from build123d import *

# Parameters (mm, degrees)
F0_W      = 50.8
F0_H      = 152.4
F1_DEPTH  = 914.4
F3_DEPTH  = 25.4
F5_DEPTH  = 914.401
F7_DEPTH  = 914.401
F9_DEPTH  = 50.801
F11_DEPTH = 27.94


with BuildPart() as f1:
    # F0 (on Right) → F1 (new body)
    with BuildSketch(Plane.YZ):
        with Locations((-25.4, 49.212513)):
            Rectangle(F0_W, F0_H)
    extrude(amount=F1_DEPTH)

    # F2 (on face) → F3 (cut)
    with BuildSketch(Plane.XZ.offset(50.8)):
        with BuildLine():
            Line((-24.162216, -26.987487), (63.5, -26.987487))
            Line((63.5, -26.987487), (63.5, 36.512513))
            ThreePointArc((63.5, 36.512513), (76.2, 49.212513), (88.9, 36.512513))
            Line((88.9, 36.512513), (88.9, -26.987487))
            Line((88.9, -26.987487), (190.5, -26.987487))
            Line((190.5, -26.987487), (190.5, 36.512513))
            ThreePointArc((190.5, 36.512513), (203.2, 49.212513), (215.9, 36.512513))
            Line((215.9, 36.512513), (215.9, -26.987487))
            Line((215.9, -26.987487), (317.5, -26.987487))
            Line((317.5, -26.987487), (317.5, 36.512513))
            ThreePointArc((317.5, 36.512513), (330.2, 49.212513), (342.9, 36.512513))
            Line((342.9, 36.512513), (342.9, -26.987487))
            Line((342.9, -26.987487), (444.5, -26.987487))
            Line((444.5, -26.987487), (444.5, 36.512513))
            ThreePointArc((444.5, 36.512513), (457.2, 49.212513), (469.9, 36.512513))
            Line((469.9, 36.512513), (469.9, -26.987487))
            Line((469.9, -26.987487), (571.5, -26.987487))
            Line((571.5, -26.987487), (571.5, 36.512513))
            ThreePointArc((571.5, 36.512513), (584.2, 49.212513), (596.9, 36.512513))
            Line((596.9, 36.512513), (596.9, -26.987487))
            Line((596.9, -26.987487), (698.5, -26.987487))
            Line((698.5, -26.987487), (698.5, 36.512513))
            ThreePointArc((698.5, 36.512513), (711.2, 49.212513), (723.9, 36.512513))
            Line((723.9, 36.512513), (723.9, -26.987487))
            Line((723.9, -26.987487), (825.5, -26.987487))
            Line((825.5, -26.987487), (825.5, 36.512513))
            ThreePointArc((825.5, 36.512513), (838.2, 49.212513), (850.9, 36.512513))
            Line((850.9, 36.512513), (850.9, -26.987487))
            Line((850.9, -26.987487), (949.602742, -26.987487))
            Line((949.602742, -26.987487), (949.602742, 67.971823))
            Line((949.602742, 67.971823), (-24.162216, 67.971823))
            Line((-24.162216, 67.971823), (-24.162216, -26.987487))
        make_face()
    extrude(amount=-F3_DEPTH, mode=Mode.SUBTRACT)

    # F4 (on Right) → F5 (cut, through all)
    with BuildSketch(Plane.YZ):
        Polygon((-50.8, -26.987487), (-24.738065, -26.987487), (-50.8, 44.617091), align=None)
    extrude(amount=F5_DEPTH, mode=Mode.SUBTRACT)

    # F6 (on Right) → F7 (cut, through all)
    with BuildSketch(Plane.YZ):
        Polygon((-50.8, 65.742032), (-29.081721, 65.742032), (-50.8, 125.412513), align=None)
    extrude(amount=F7_DEPTH, mode=Mode.SUBTRACT)

    # F8 (on Front) → F9 (cut, through all)
    with BuildSketch(Plane.XZ):
        with BuildLine():
            Line((-17.833117, 74.612513), (0, 74.612513))
            Line((0, 74.612513), (0, 112.712513))
            ThreePointArc((0, 112.712513), (12.7, 125.412513), (25.4, 112.712513))
            Line((25.4, 112.712513), (25.4, 74.612513))
            Line((25.4, 74.612513), (127, 74.612513))
            Line((127, 74.612513), (127, 112.712513))
            ThreePointArc((127, 112.712513), (139.7, 125.412513), (152.4, 112.712513))
            Line((152.4, 112.712513), (152.4, 74.612513))
            Line((152.4, 74.612513), (254, 74.612513))
            Line((254, 74.612513), (254, 112.712513))
            ThreePointArc((254, 112.712513), (266.7, 125.412513), (279.4, 112.712513))
            Line((279.4, 112.712513), (279.4, 74.612513))
            Line((279.4, 74.612513), (381, 74.612513))
            Line((381, 74.612513), (381, 112.712513))
            ThreePointArc((381, 112.712513), (393.7, 125.412513), (406.4, 112.712513))
            Line((406.4, 112.712513), (406.4, 74.612513))
            Line((406.4, 74.612513), (508, 74.612513))
            Line((508, 74.612513), (508, 112.712513))
            ThreePointArc((508, 112.712513), (520.7, 125.412513), (533.4, 112.712513))
            Line((533.4, 112.712513), (533.4, 74.612513))
            Line((533.4, 74.612513), (635, 74.612513))
            Line((635, 74.612513), (635, 112.712513))
            ThreePointArc((635, 112.712513), (647.7, 125.412513), (660.4, 112.712513))
            Line((660.4, 112.712513), (660.4, 74.612513))
            Line((660.4, 74.612513), (762, 74.612513))
            Line((762, 74.612513), (762, 112.712513))
            ThreePointArc((762, 112.712513), (774.7, 125.412513), (787.4, 112.712513))
            Line((787.4, 112.712513), (787.4, 74.612513))
            Line((787.4, 74.612513), (889, 74.612513))
            Line((889, 74.612513), (889, 112.712513))
            ThreePointArc((889, 112.712513), (901.7, 125.412513), (914.4, 112.712513))
            Line((914.4, 112.712513), (914.4, 74.612513))
            Line((914.4, 74.612513), (957.003824, 74.612513))
            Line((957.003824, 74.612513), (957.003824, 229.980152))
            Line((957.003824, 229.980152), (-17.833117, 229.980152))
            Line((-17.833117, 229.980152), (-17.833117, 74.612513))
        make_face()
    extrude(amount=F9_DEPTH, mode=Mode.SUBTRACT)

    # F10 (on face) → F11 (cut)
    with BuildSketch(Plane(origin=(0, 0, 0), x_dir=(-1, 0, 0), z_dir=(0, 1, 0))):
        with BuildLine():
            Line((-806.45, 112.712513), (-869.95, 112.712513))
            ThreePointArc((-869.95, 112.712513), (-874.440128, 110.852641), (-876.3, 106.362513))
            Line((-876.3, 106.362513), (-876.3, 17.462513))
            ThreePointArc((-876.3, 17.462513), (-874.440128, 12.972385), (-869.95, 11.112513))
            Line((-869.95, 11.112513), (-806.45, 11.112513))
            ThreePointArc((-806.45, 11.112513), (-801.959872, 12.972385), (-800.1, 17.462513))
            Line((-800.1, 17.462513), (-800.1, 106.362513))
            ThreePointArc((-800.1, 106.362513), (-801.959872, 110.852641), (-806.45, 112.712513))
        make_face()
        with BuildLine():
            Line((-679.45, 112.712513), (-742.95, 112.712513))
            ThreePointArc((-742.95, 112.712513), (-747.440128, 110.852641), (-749.3, 106.362513))
            Line((-749.3, 106.362513), (-749.3, 17.462513))
            ThreePointArc((-749.3, 17.462513), (-747.440128, 12.972385), (-742.95, 11.112513))
            Line((-742.95, 11.112513), (-679.45, 11.112513))
            ThreePointArc((-679.45, 11.112513), (-674.959872, 12.972385), (-673.1, 17.462513))
            Line((-673.1, 17.462513), (-673.1, 106.362513))
            ThreePointArc((-673.1, 106.362513), (-674.959872, 110.852641), (-679.45, 112.712513))
        make_face()
        with BuildLine():
            Line((-552.45, 112.712513), (-615.95, 112.712513))
            ThreePointArc((-615.95, 112.712513), (-620.440128, 110.852641), (-622.3, 106.362513))
            Line((-622.3, 106.362513), (-622.3, 17.462513))
            ThreePointArc((-622.3, 17.462513), (-620.440128, 12.972385), (-615.95, 11.112513))
            Line((-615.95, 11.112513), (-552.45, 11.112513))
            ThreePointArc((-552.45, 11.112513), (-547.959872, 12.972385), (-546.1, 17.462513))
            Line((-546.1, 17.462513), (-546.1, 106.362513))
            ThreePointArc((-546.1, 106.362513), (-547.959872, 110.852641), (-552.45, 112.712513))
        make_face()
        with BuildLine():
            Line((-425.45, 112.712513), (-488.95, 112.712513))
            ThreePointArc((-488.95, 112.712513), (-493.440128, 110.852641), (-495.3, 106.362513))
            Line((-495.3, 106.362513), (-495.3, 17.462513))
            ThreePointArc((-495.3, 17.462513), (-493.440128, 12.972385), (-488.95, 11.112513))
            Line((-488.95, 11.112513), (-425.45, 11.112513))
            ThreePointArc((-425.45, 11.112513), (-420.959872, 12.972385), (-419.1, 17.462513))
            Line((-419.1, 17.462513), (-419.1, 106.362513))
            ThreePointArc((-419.1, 106.362513), (-420.959872, 110.852641), (-425.45, 112.712513))
        make_face()
        with BuildLine():
            Line((-298.45, 112.712513), (-361.95, 112.712513))
            ThreePointArc((-361.95, 112.712513), (-366.440128, 110.852641), (-368.3, 106.362513))
            Line((-368.3, 106.362513), (-368.3, 17.462513))
            ThreePointArc((-368.3, 17.462513), (-366.440128, 12.972385), (-361.95, 11.112513))
            Line((-361.95, 11.112513), (-298.45, 11.112513))
            ThreePointArc((-298.45, 11.112513), (-293.959872, 12.972385), (-292.1, 17.462513))
            Line((-292.1, 17.462513), (-292.1, 106.362513))
            ThreePointArc((-292.1, 106.362513), (-293.959872, 110.852641), (-298.45, 112.712513))
        make_face()
        with BuildLine():
            Line((-171.45, 112.712513), (-234.95, 112.712513))
            ThreePointArc((-234.95, 112.712513), (-239.440128, 110.852641), (-241.3, 106.362513))
            Line((-241.3, 106.362513), (-241.3, 17.462513))
            ThreePointArc((-241.3, 17.462513), (-239.440128, 12.972385), (-234.95, 11.112513))
            Line((-234.95, 11.112513), (-171.45, 11.112513))
            ThreePointArc((-171.45, 11.112513), (-166.959872, 12.972385), (-165.1, 17.462513))
            Line((-165.1, 17.462513), (-165.1, 106.362513))
            ThreePointArc((-165.1, 106.362513), (-166.959872, 110.852641), (-171.45, 112.712513))
        make_face()
        with BuildLine():
            Line((-44.45, 112.712513), (-107.95, 112.712513))
            ThreePointArc((-107.95, 112.712513), (-112.440128, 110.852641), (-114.3, 106.362513))
            Line((-114.3, 106.362513), (-114.3, 17.462513))
            ThreePointArc((-114.3, 17.462513), (-112.440128, 12.972385), (-107.95, 11.112513))
            Line((-107.95, 11.112513), (-44.45, 11.112513))
            ThreePointArc((-44.45, 11.112513), (-39.959872, 12.972385), (-38.1, 17.462513))
            Line((-38.1, 17.462513), (-38.1, 106.362513))
            ThreePointArc((-38.1, 106.362513), (-39.959872, 110.852641), (-44.45, 112.712513))
        make_face()
    extrude(amount=-F11_DEPTH, mode=Mode.SUBTRACT)


solid = f1.part
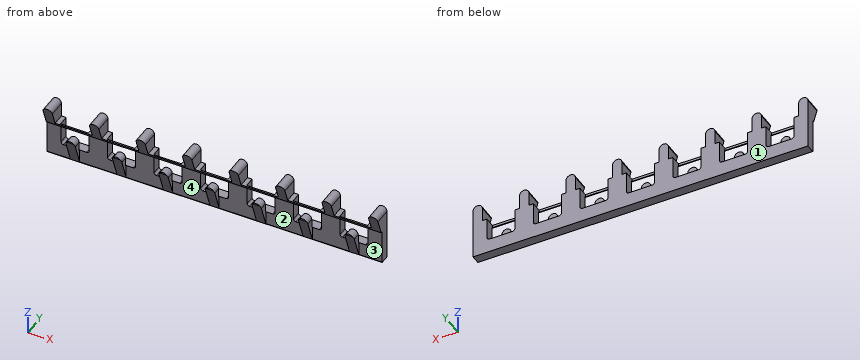
Check sheet for the modelled part. Datum: model origin and axes. Units: mm. Face numbers are marked on the shaded views. A direction names the side the tool comes from. Round coordinates to 2 decimals unless told otherwise and drop trailing zeros. Order: outer loops, then holes, each group sorted by start corner. A loop starts at its lowest first (then second) coordinate and runs counter-clockwise, first axis right, second up.
(1) Draft check along X on the marked faces 3 and 4. Enter one of: pulls with the +X half, pulls with the -X half, needs draft (parallel to the pull), parting line crosses it, or undercut.
(2) Go/stop test with flat-tipped pins: P1, Ø9.5, axis at x = 341.5, y = -9.5, coming from the +Z side; P2, Ø8, axis at y = -33.5, z = 44, coming from the +X side; P3, Ø10, axis at x = 232, y = -15.5, coming from the +Z side; P4, Ø2, axis at y = -35, z = 76.5, coming from the -X side. Record where each tip stops, or that it passes through.
(3) Cross-section at C-C, the plane x = 838.2. Enter the section's corners in (y, z).
(4) Cross-section at D-D, the plane x = 201. Enter the section's corners in (y, z).
(5) Access from +Z, -Z, +X, -X, +Y, -Y to the whole of each face (thin tool, end or side, straight path). Record for the marked faces 1 and 2.
(6) Scan lines: probe 1 along Z at (x, y) = (562.5, -7.5); probe 2 along Y at (x, z) = (528.5, 34); probe 3 along Z at (x, y) = (752.5, -18). Record each from-to range of solid material in increasing order.
(7) Cross-section at B-B, the plane z = 104.5. State how many separate pieces and enclosed holes the cut face has, and give its area (3 significant figures).
(8) Cross-section at A-A, the plane x = 479.5. Enter the section's corners in (y, z).
Check sheet entries:
1. face 3: needs draft
1. face 4: undercut
2. P1: stops at z = 11.11
2. P2: stops at x = 850.41
2. P3: stops at z = 11.45
2. P4: passes through
3. outline: (-50.8, 44.62) - (-24.74, -26.99) - (0, -26.99) - (0, 11.11) - (-27.94, 11.11) - (-27.94, 49.21) - (-50.8, 49.21) - close; (-32.31, 74.61) - (-29.89, 67.97) - (-27.94, 67.97) - (-27.94, 74.61) - close
4. outline: (-50.8, 44.62) - (-24.74, -26.99) - (0, -26.99) - (0, 11.11) - (-27.94, 11.11) - (-27.94, 49.02) - (-50.8, 49.02) - close; (-32.31, 74.61) - (-29.89, 67.97) - (-27.94, 67.97) - (-27.94, 74.61) - close
5. face 1: +Z, -Z, +X, -X, +Y
5. face 2: -Z, -Y
6. probe 1: z = -26.99 to 11.11
6. probe 2: y = -25.4 to 0
6. probe 3: z = -26.99 to 74.61
7. separate pieces: 8
7. enclosed holes: 0
7. area: 8,780 mm2
8. outline: (-32.31, 74.61) - (-29.89, 67.97) - (-27.94, 67.97) - (-27.94, 74.61) - close; (-25.4, -25.17) - (-24.74, -26.99) - (0, -26.99) - (0, 11.11) - (-25.4, 11.11) - close
